Study the drawing (mm; zero at the part's minimum x, y, z) and answer. A direction names the side the tool comes from. Coordinates: 2 decimals unless noted, no trailing zeros. Order: outer loops, then holes, each group sorted by start corner. A loop starts at its lowest first (then second) coordinate and runs counter-clockwise, first axis right, second up.
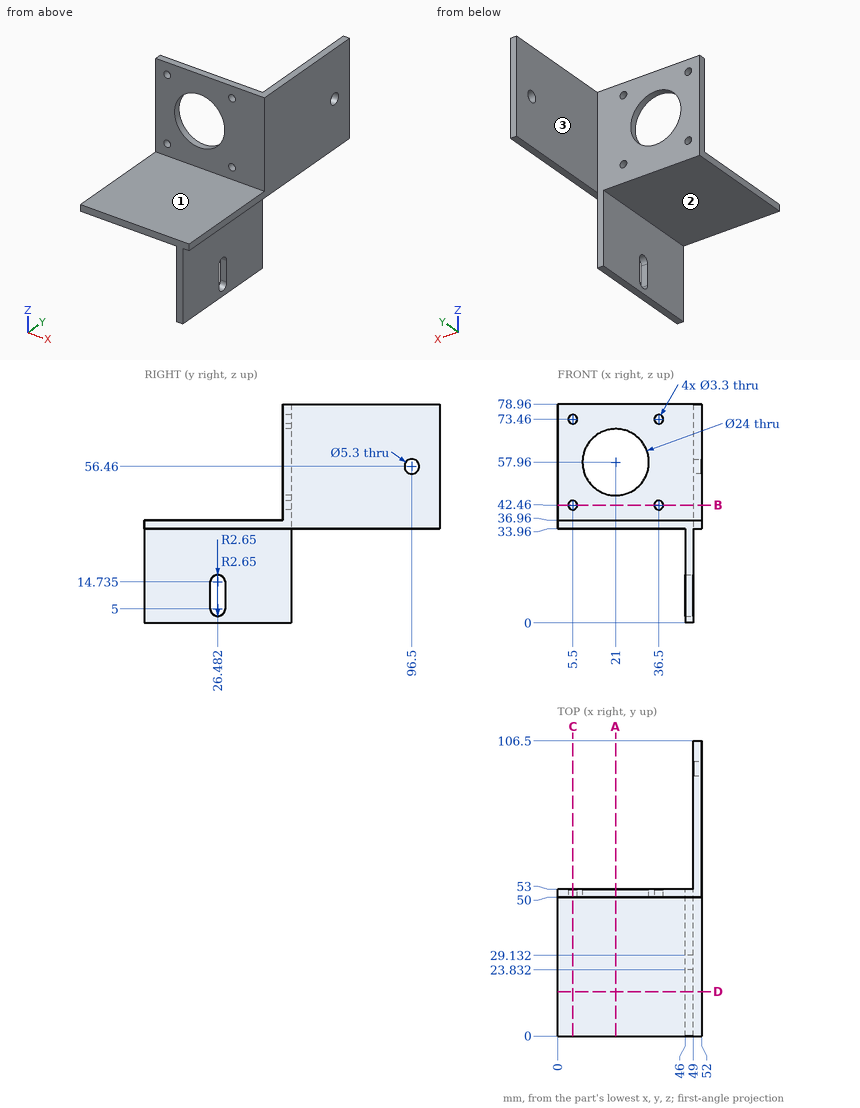
1) A cutting plane is placed at C-C, the plane x = 5.5. Determine the outline of the cut face in (y, z), and give its area (3 significant figures).
A:
outline: (0, 33.96) - (53, 33.96) - (53, 40.81) - (50, 40.81) - (50, 36.96) - (0, 36.96) - close; (50, 44.11) - (53, 44.11) - (53, 71.81) - (50, 71.81) - close; (50, 75.11) - (53, 75.11) - (53, 78.96) - (50, 78.96) - close
area: 265 mm2
2) Flat-ended cylindrical pins translate along their axes: pin 1 Ø1 at (y, z) = (21, 28.5) entering from -X; pin 2 Ø1.5 at (x, z) = (47.5, 9) entering from +Y; pin 3 Ø0.9 at (x, y) = (50.5, 70) entering from -Z. Find the tip coordinate at first contact, or state that the pin passes through.
A:
pin 1: stops at x = 46
pin 2: stops at y = 53
pin 3: stops at z = 33.96
3) A cutting plane is placed at B-B, the plane z = 42.46. Determine the outline of the cut face in (x, y), and give its area (3 significant figures).
A:
outline: (0, 50) - (3.85, 50) - (3.85, 53) - (0, 53) - close; (7.15, 50) - (34.85, 50) - (34.85, 53) - (7.15, 53) - close; (38.15, 50) - (52, 50) - (52, 106.5) - (49, 106.5) - (49, 53) - (38.15, 53) - close
area: 297 mm2
4) Straight lines are drawn through the part: line 1 (Z direction, x = 36.5, y = 50.95); line 2 (Z direction, x = 49.75, y = 96.5); line 3 (Y direction, x = 50.95, z = 56.46). For each, find the intervals that lie inside material, in ascending order.
A:
line 1: z = 33.96 to 40.81, 44.11 to 71.81, 75.11 to 78.96
line 2: z = 33.96 to 53.81, 59.11 to 78.96
line 3: y = 50 to 93.85, 99.15 to 106.5
5) A cutting plane is placed at D-D, the plane y = 16. Determine the outline of the cut face in (x, z), and give its area (3 significant figures).
A:
outline: (0, 33.96) - (46, 33.96) - (46, 0) - (49, 0) - (49, 33.96) - (52, 33.96) - (52, 36.96) - (0, 36.96) - close
area: 258 mm2
6) A cutting plane is placed at A-A, the plane x = 21. Determine the outline of the cut face in (y, z).
A:
outline: (0, 33.96) - (53, 33.96) - (53, 45.96) - (50, 45.96) - (50, 36.96) - (0, 36.96) - close; (50, 69.96) - (53, 69.96) - (53, 78.96) - (50, 78.96) - close
7) Which of the six approach directions +Z, -Z, +X, -X, +Y, -Y give full straight-line access (tool end or side, diameter ignored) to the marked faces 1, 2 and 3?
A:
face 1: +Z, +X, -X, -Y
face 2: -Z, -X, +Y, -Y
face 3: +Z, -Z, -X, +Y
